Model file for the job. Use its own axes, mm. Face numbers are marked on the shaded views. A direction names the side the tool comes from. Round coordinates to 2 decimals unless told otherwise and drop trailing zeros. Order: outer loops, then holes, each group sorted by start corner. A loop starts at its lowest first (then second) coordinate and runs counter-clockwise, first axis right, second up. Notation, with made-up numbers: (35, 45.25) - (88, 45.25) arc R13 ccw to (88, 50.25) - close; hole circle Ø6 at (7, 45.5). An arc over 180 degrees is marked (long way). Use one line per item in the form item = value.
from build123d import *

# Parameters (mm, degrees)
SKETCH_1_W        = 28.7
SKETCH_1_H        = 26.7
SKETCH_1_W_2      = 25.7
SKETCH_1_H_2      = 23.7
EXTRUDE_2_DEPTH   = 2
SKETCH_1_7_R      = 3
SKETCH_1_7_R_2    = 1.1
EXTRUDE_5_DEPTH   = 5
EXTRUDE_5_2_DEPTH = 5
SKETCH_1_8_W      = 47
SKETCH_1_8_H      = 43
EXTRUDE_6_DEPTH   = 5


with BuildPart() as part:
    # Sketch 1 → Extrude 2 (new body)
    with BuildSketch(Plane.XY):
        Rectangle(SKETCH_1_W, SKETCH_1_H)
        Rectangle(SKETCH_1_W_2, SKETCH_1_H_2, mode=Mode.SUBTRACT)
    extrude(amount=EXTRUDE_2_DEPTH)



with BuildPart() as body_2:
    # Sketch 1_7 → Extrude 5 (new body)
    with BuildSketch(Plane.XY):
        with Locations((17.5, 0)):
            Circle(SKETCH_1_7_R)
        with Locations((17.5, 0)):
            Circle(SKETCH_1_7_R_2, mode=Mode.SUBTRACT)
    extrude(amount=EXTRUDE_5_DEPTH)


with BuildPart() as body_3:
    # Sketch 1_7 → Extrude 5 2 (new body)
    with BuildSketch(Plane.XY):
        with Locations((-17.5, 0)):
            Circle(SKETCH_1_7_R)
        with Locations((-17.5, 0)):
            Circle(SKETCH_1_7_R_2, mode=Mode.SUBTRACT)
    extrude(amount=EXTRUDE_5_2_DEPTH)


with BuildPart() as part_1:
    add(part.part)

    add(body_2.part)  # Extrude 6 merges body 2

    add(body_3.part)  # Extrude 6 merges body 3
    # Sketch 1_8 → Extrude 6 (add)
    with BuildSketch(Plane.XY):
        Rectangle(SKETCH_1_8_W, SKETCH_1_8_H)
    extrude(amount=-EXTRUDE_6_DEPTH)


solid = part_1.part
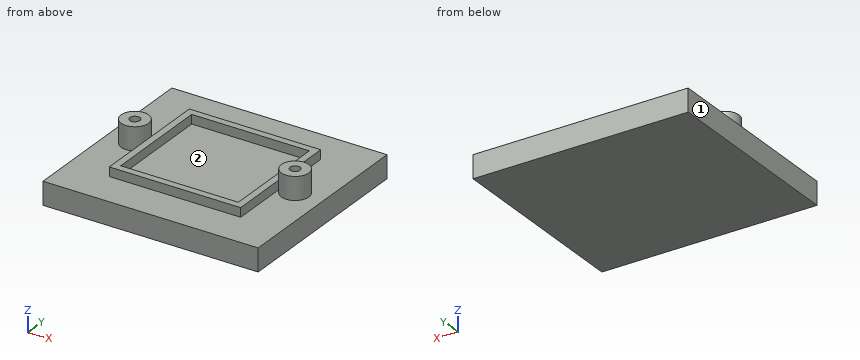
(1) Slice it at D-D on x = -17.5. Give the cut face in (y, z), then the cut area to 3 significant figures.
Report:
outline = (-21.5, -5) - (21.5, -5) - (21.5, 0) - (3, 0) - (3, 5) - (1.1, 5) - (1.1, 0) - (-1.1, 0) - (-1.1, 5) - (-3, 5) - (-3, 0) - (-21.5, 0) - close
area = 234 mm2
(2) Slice it at C-C on y = 0. Give the cut face in (x, z).
Report:
outline = (-23.5, -5) - (23.5, -5) - (23.5, 0) - (20.5, 0) - (20.5, 5) - (18.6, 5) - (18.6, 0) - (16.4, 0) - (16.4, 5) - (14.5, 5) - (14.5, 0) - (14.35, 0) - (14.35, 2) - (12.85, 2) - (12.85, 0) - (-12.85, 0) - (-12.85, 2) - (-14.35, 2) - (-14.35, 0) - (-14.5, 0) - (-14.5, 5) - (-16.4, 5) - (-16.4, 0) - (-18.6, 0) - (-18.6, 5) - (-20.5, 5) - (-20.5, 0) - (-23.5, 0) - close
(3) Slice it at B-B on x = 5. Give the cut face in (y, z).
Report:
outline = (-21.5, -5) - (21.5, -5) - (21.5, 0) - (13.35, 0) - (13.35, 2) - (11.85, 2) - (11.85, 0) - (-11.85, 0) - (-11.85, 2) - (-13.35, 2) - (-13.35, 0) - (-21.5, 0) - close
(4) Slice it at A-A on z = 0.75. Give the cut face in (x, y).
Report:
outline = circle Ø6 at (-17.5, 0); (-14.35, -13.35) - (14.35, -13.35) - (14.35, 13.35) - (-14.35, 13.35) - close; circle Ø6 at (17.5, 0); hole circle Ø2.2 at (-17.5, 0); hole (-12.85, -11.85) - (12.85, -11.85) - (12.85, 11.85) - (-12.85, 11.85) - close; hole circle Ø2.2 at (17.5, 0)
(5) Pin check, flat tips, straight feed: pin 1 (21.5 mm diameter, centred on x = 3, y = 5, fed in from +Z); pin 2 (2 mm diameter, centred on x = 2.5, z = 1.5, fed in from +Y); pin 3 (0.6 mm diameter, centred on y = -4.5, z = 1, fed in from -X). Stop position of each tip, or through.
Report:
pin_1 = 2
pin_2 = 13.35
pin_3 = -14.35
(6) Tool access for the marked faces 1 and 2: list every direction of +Z, -Z, +X, -X, +Y, -Y with a clear straight run to the whole face (end or side of a thin tool).
Report:
face_1 = +Z, -Z, -X, +Y, -Y
face_2 = +Z
(7) Probe probe 1 along Y at (x, z) = (17.5, 2.7); probe 2 along Z at (x, y) = (2, -4); probe 3 along Z at (x, y) = (13, 8). List the from-to ranges inside material, lowest first. Write a range as [from, to].
Report:
probe_1 = [-3, -1.1], [1.1, 3]
probe_2 = [-5, 0]
probe_3 = [-5, 2]
